Can you work these out from the drawing? Everything is in mm from the part's minimum corner. Round coordinates to 2 decimals unless told otherwise and drop trailing zeros. Write each loop counter-clockwise with the first axis right and the second up, starting at its lowest first coordinate (ties: lowest second). Pieces come first, ordered by that corner, then holes. Notation, with made-up numbers: M 8.25,36.25 L 23.25,36.25 A16 ccw 23.25,56.25 Z; hole C 87.25,59.5 d10. An arc over 180 degrees is marked long. Answer in a Markdown table with one row per item. Add a question column.
(1) Suppose I cut it at B-B, the plane y = 13. Write out the boundary of the cut face in (x, z).
(2) If I drill on probe 1 along Z at (x, y) = (11.5, 2.25); probe 2 along Y at (x, z) = (19.75, 33) (1 decimal); probe 3 along X at (y, z) = (7.75, 38) (1 decimal), over which ranges is the centre line in solid material (lowest first)?
(3) If we mould it in two halves opening along X, with no side actions, what happens to the marked faces 1, 2 and 3? For each: released by +X, released by -X, zero draft, split by the parting line, or undercut.
(4) I'm going to push flat-ended pins straight in: pin 1 (10 mm diameter, centred on y = 21, z = 12.5, fed in from -X); pin 2 (1 mm diameter, centred on x = 4.5, z = 21.5, fed in from +Y) (1 decimal); pin 3 (3 mm diameter, centred on x = 13.53, y = 13.53, fed in from +Z); pin 4 (1 mm diameter, centred on y = 15, z = 27, fed in from +X). Where does each tip first touch, or does it pass through?
(5) Suppose I cut it at C-C, the plane z = 5. Count the separate pieces of the cut face and the enclosed holes in it.
(6) Suppose I cut it at D-D, the plane y = 2. Write out the boundary of the cut face in (x, z).
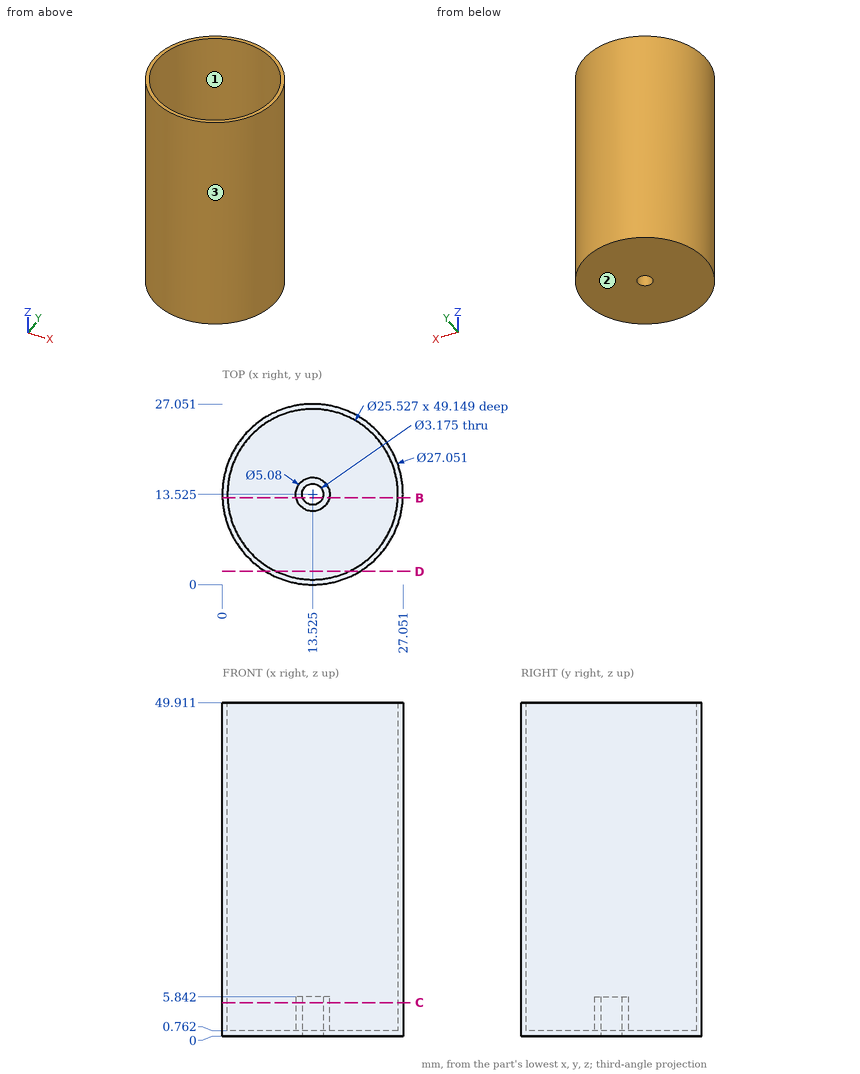
Calculated:
| question | item | result |
|---|---|---|
| 1 | outline | M 0.01,0 L 12.03,0 L 12.03,5.84 L 11.04,5.84 L 11.04,0.76 L 0.77,0.76 L 0.77,49.91 L 0.01,49.91 Z; M 15.02,0 L 27.04,0 L 27.04,49.91 L 26.28,49.91 L 26.28,0.76 L 16.01,0.76 L 16.01,5.84 L 15.02,5.84 Z |
| 2 | probe 1 | 0 to 0.76 |
| 2 | probe 2 | 1.5 to 2.4, 24.7 to 25.5 |
| 2 | probe 3 | 1.3 to 2.1, 24.9 to 25.8 |
| 3 | face 1 | undercut |
| 3 | face 2 | zero draft |
| 3 | face 3 | split by the parting line |
| 4 | pin 1 | x = 0.23 |
| 4 | pin 2 | y = 24 |
| 4 | pin 3 | through |
| 4 | pin 4 | x = 27.02 |
| 5 | separate pieces | 2 |
| 5 | enclosed holes | 2 |
| 6 | outline | M 6.45,0 L 20.6,0 L 20.6,49.91 L 19.01,49.91 L 19.01,0.76 L 8.04,0.76 L 8.04,49.91 L 6.45,49.91 Z |
